Could you check a few things on this model? Use its own coordinates, in mm. Round coordinates to 2 decimals unless told otherwise and drop trailing zeros. Loops run counter-clockwise (first coordinate to the right, second up) from the corner with the lowest first, then second, coordinate; pieces in that order, holes last.
from build123d import *

# Parameters (mm, degrees)
BOSS_EXTRUDE1_DEPTH = 6
CUT_EXTRUDE1_DEPTH  = 779.722672073
FILLET1_R           = 2
SKETCH4_W           = 56.4
SKETCH4_H           = 6
CUT_EXTRUDE4_DEPTH  = 1


with BuildPart() as part:
    # Sketch1 → Boss-Extrude1 (new body)
    with BuildSketch(Plane(origin=(0, 0, 0.563566935), x_dir=(-1, 0, 0), z_dir=(0, 0, -1))):
        with BuildLine():
            Line((29.2, 33), (-29.2, 33))
            Line((-29.2, 33), (-29.2, 20))
            Line((-29.2, 20), (-770.043194655, 15.999883388))
            ThreePointArc((-770.043194655, 15.999883388), (-777.999970847, 7.978402594), (-770, 0))
            Line((-770, 0), (770, 0))
            ThreePointArc((770, 0), (777.999970847, 7.978402594), (770.043194655, 15.999883388))
            Line((770.043194655, 15.999883388), (29.2, 20))
            Line((29.2, 20), (29.2, 33))
        make_face()
    extrude(amount=-BOSS_EXTRUDE1_DEPTH)

    # Sketch2 → Cut-Extrude1 (cut, through all)
    with BuildSketch(Plane(origin=(0, 0, 0.563566935), x_dir=(-1, 0, 0), z_dir=(0, 0, -1))):
        with BuildLine():
            Line((28.2, 19.005384834), (28.2, 32))
            Line((28.2, 32), (-28.2, 32))
            Line((-28.2, 32), (-28.2, 19.005384834))
            Line((-28.2, 19.005384834), (-770.037795323, 14.999897965))
            ThreePointArc((-770.037795323, 14.999897965), (-776.999974491, 7.981102269), (-770, 1))
            Line((-770, 1), (770, 1))
            ThreePointArc((770, 1), (776.999974491, 7.981102269), (770.037795323, 14.999897965))
            Line((770.037795323, 14.999897965), (28.2, 19.005384834))
        make_face()
    extrude(amount=-CUT_EXTRUDE1_DEPTH, mode=Mode.SUBTRACT)

    # Fillet1
    fillet1_edges = [part.edges().sort_by_distance(p)[0] for p in [
        (-29.2, 20, 3.563566935),
        (29.2, 20, 3.563566935),
        (-28.2, 19.005384834, 3.563566935),
        (28.2, 19.005384834, 3.563566935),
    ]]
    fillet(fillet1_edges, radius=FILLET1_R)

    # Sketch4 → Cut-Extrude4 (cut)
    with BuildSketch(Plane(origin=(0, 33, 0), x_dir=(-1, 0, 0), z_dir=(0, 1, 0))):
        with Locations((0, 3.563566935)):
            Rectangle(SKETCH4_W, SKETCH4_H)
    extrude(amount=-CUT_EXTRUDE4_DEPTH, mode=Mode.SUBTRACT)


solid = part.part
Item 1: If we section it at B-B, the plane z = 5.5: Please give me the cut outline in (x, y), then the cut area to 3 significant figures.
Results list:
outline: (-770.04, 15) - (-30.19, 18.99) arc R2 ccw to (-28.2, 20.99) - (-28.2, 33) - (-29.2, 33) - (-29.2, 21.99) arc R2 cw to (-31.19, 19.99) - (-770.04, 16) arc R8 ccw to (-770, 0) - (770, 0) arc R8 ccw to (770.04, 16) - (31.19, 19.99) arc R2 cw to (29.2, 21.99) - (29.2, 33) - (28.2, 33) - (28.2, 20.99) arc R2 ccw to (30.19, 18.99) - (770.04, 15) arc R7 cw to (770, 1) - (-770, 1) arc R7 cw to start
area: 3,100 mm2
Item 2: If we section it at A-A, the plane y = 8: Please give me the cut outline in (x, z), then the cut area to 3 significant figures.
Results list:
outline: (-778, 0.56) - (-777, 0.56) - (-777, 6.56) - (-778, 6.56) - close; (777, 0.56) - (778, 0.56) - (778, 6.56) - (777, 6.56) - close
area: 12.0 mm2
Item 3: If I drill on line 1 along Y through (x, z) = (75, 1.5); line 2 along X through (y, z) = (23, 5); line 3 along X through (y, z) = (9, 5), over which ranges is the centre line in solid material (lowest first)?
Results list:
line 1: y = 0 to 1, 18.75 to 19.75
line 2: x = -29.2 to -28.2, 28.2 to 29.2
line 3: x = -777.94 to -776.93, 776.93 to 777.94
Item 4: If we section it at C-C, the plane x = -195: Please give me the cut outline in (y, z).
Results list:
outline: (0, 0.56) - (1, 0.56) - (1, 6.56) - (0, 6.56) - close; (18.1, 0.56) - (19.1, 0.56) - (19.1, 6.56) - (18.1, 6.56) - close
Item 5: Will these pins go through, and if not, where does the flat tip stop? pin 1 (3 mm diameter, centred on y = 25, z = 5, fed in from -X); pin 2 (5 mm diameter, centred on x = -34, y = 22, fed in from -Z); pin 3 (1.8 mm diameter, centred on y = 29.5, z = 3, fed in from +X).
Results list:
pin 1: stops at x = -29.2
pin 2: stops at z = 0.56
pin 3: stops at x = 29.2
